Verification items for the finished model (mm, model axes). A direction names the side the tool comes from. Round coordinates to 2 decimals unless told otherwise and drop trailing zeros. Write each loop counter-clockwise with the first axis right and the second up, starting at its lowest first coordinate (ties: lowest second). Pieces come first, ordered by that corner, then holes. Notation, with made-up numbers: M 32,50.5 L 45,50.5 A23 ccw 45,69.5 Z; hole C -21.5,78.5 d6. An arc over 180 degrees is marked long. One line per question, with ' | ' between items. Start each with the question number.
Q1. Cross-section at B-B (y = -9.25). Record the boundary of the cut face in (x, z), then the cut area to 3 significant figures.
Q2. Tool access check on faces 1 (the face through (10.5, -6, 52)), 2 (the face through (-12, -5, 4)), 3 (the face through (-14, -3.5, 67)). Record the directions out of +Z, -Z, +X, -X, +Y, -Y that give a thin tool (end or side, any length) a straight path to the whole face; none if there is none.
Q3. Cross-section at A-A (x = -3.5). Record the boundary of the cut face in (y, z), then the cut area to 3 significant figures.
Q4. Gauge pin test, flat ends, axial feed: pin 1 (10 mm diameter, centred on x = 7, z = 36.5, fed in from -Y); pin 2 (4 mm diameter, centred on x = 1, z = 97, fed in from +Y); pin 3 (6 mm diameter, centred on x = -5.5, y = 9.5, fed in from +Z). Record the tip position at first contact, or that the pin passes through.
Q5. Thickness scan on line 1 along Y through (x, z) = (-10, 24); line 2 along Z through (x, y) = (7.25, 3.5); line 3 along X through (y, z) = (-6.5, 30). Record the ranges inside material, lowest first. Write a range as from..to.
from build123d import *

# Parameters (mm, degrees)
CROQUIS1_W              = 29
CROQUIS1_H              = 18
SALIENTE_EXTRUIR1_DEPTH = 4
CROQUIS2_W              = 6
CROQUIS2_H              = 4
CROQUIS2_W_2            = 9
SALIENTE_EXTRUIR3_DEPTH = 4
CROQUIS4_W              = 4.5
CROQUIS4_H              = 4
SALIENTE_EXTRUIR4_DEPTH = 100
CROQUIS5_W              = 7
CROQUIS5_H              = 4
SALIENTE_EXTRUIR5_DEPTH = 100
CROQUIS6_W              = 30
CROQUIS6_H              = 4
SALIENTE_EXTRUIR6_DEPTH = 10
CORTAR_EXTRUIR2_DEPTH   = 10
CORTAR_EXTRUIR3_DEPTH   = 10
CORTAR_EXTRUIR4_DEPTH   = 10
CORTAR_EXTRUIR5_DEPTH   = 10


with BuildPart() as part:
    # Croquis1 → Saliente-Extruir1 (new body)
    with BuildSketch(Plane(origin=(0, 0, 0), x_dir=(0, 1, 0), z_dir=(0, 0, 1))):
        Rectangle(CROQUIS1_W, CROQUIS1_H)
    extrude(amount=SALIENTE_EXTRUIR1_DEPTH)

    # Croquis2 → Saliente-Extruir3 (add)
    with BuildSketch(Plane.XY.offset(4)):
        with Locations((-12, -5.5)):
            Rectangle(CROQUIS2_W, CROQUIS2_H)
        with Locations((-4.5, -5.5)):
            Rectangle(CROQUIS2_W_2, CROQUIS2_H)
        with Locations((4.5, -5.5)):
            Rectangle(CROQUIS2_W_2, CROQUIS2_H)
        with Locations((12, -5.5)):
            Rectangle(CROQUIS2_W, CROQUIS2_H)
    extrude(amount=SALIENTE_EXTRUIR3_DEPTH)

    # Croquis4 → Saliente-Extruir4 (add)
    with BuildSketch(Plane.XY.offset(8)):
        with Locations((12.75, -5.5)):
            Rectangle(CROQUIS4_W, CROQUIS4_H)
    extrude(amount=SALIENTE_EXTRUIR4_DEPTH)

    # Croquis5 → Saliente-Extruir5 (add)
    with BuildSketch(Plane.XY.offset(8)):
        with Locations((-11.5, -5.5)):
            Rectangle(CROQUIS5_W, CROQUIS5_H)
    extrude(amount=SALIENTE_EXTRUIR5_DEPTH)

    # Croquis6 → Saliente-Extruir6 (add)
    with BuildSketch(Plane.XY.offset(108)):
        with Locations((0, -5.5)):
            Rectangle(CROQUIS6_W, CROQUIS6_H)
    extrude(amount=-SALIENTE_EXTRUIR6_DEPTH)

    # Croquis7 → Cortar-Extruir2 (cut)
    with BuildSketch(Plane.XZ.offset(7.5)):
        Polygon((-8, 96.258476268), (-8, 97.519571135), (-11.46482967, 97.519571135), align=None)
    extrude(amount=-CORTAR_EXTRUIR2_DEPTH, mode=Mode.SUBTRACT)

    # Croquis8 → Cortar-Extruir3 (cut)
    with BuildSketch(Plane(origin=(0, -7.5, 0), x_dir=(-1, 0, 0), z_dir=(0, -1, 0))):
        Polygon((8, -94.994476268), (11.46482967, -93.733381401), (8, -93.733381401), align=None)
    extrude(amount=-CORTAR_EXTRUIR3_DEPTH, mode=Mode.SUBTRACT)

    # Croquis9 → Cortar-Extruir4 (cut)
    with BuildSketch(Plane(origin=(0, -7.5, 0), x_dir=(-1, 0, 0), z_dir=(0, -1, 0))):
        Polygon((11.46482967, -93.733381401), (11.46482967, -92.469381401), (8, -91.208286534), (8, -93.733381401), align=None)
    extrude(amount=-CORTAR_EXTRUIR4_DEPTH, mode=Mode.SUBTRACT)

    # Croquis10 → Cortar-Extruir5 (cut)
    with BuildSketch(Plane(origin=(0, -3.5, 0), x_dir=(-1, 0, 0), z_dir=(0, 1, 0))):
        Polygon((11.46482967, 11.070269037), (8, 9.80917417), (8, 13.595363904), (11.46482967, 12.334269037), align=None)
        Polygon((11.46482967, 88.087115043), (8, 89.348209909), (8, 85.562020176), (11.46482967, 86.823115043), align=None)
        Polygon((8, 84.298020176), (11.46482967, 83.036925309), (11.46482967, 81.772925309), (8, 80.511830442), align=None)
        Polygon((8, 79.247830442), (11.46482967, 77.986735575), (11.46482967, 76.722735575), (8, 75.461640708), align=None)
        Polygon((8, 70.411450974), (8, 74.197640708), (11.46482967, 72.936545841), (11.46482967, 71.672545841), align=None)
        Polygon((8, 65.361261241), (8, 69.147450974), (11.46482967, 67.886356108), (11.46482967, 66.622356108), align=None)
        Polygon((8, 60.311071507), (8, 64.097261241), (11.46482967, 62.836166374), (11.46482967, 61.572166374), align=None)
        Polygon((8, 55.260881773), (8, 59.047071507), (11.46482967, 57.78597664), (11.46482967, 56.52197664), align=None)
        Polygon((8, 50.21069204), (8, 53.996881773), (11.46482967, 52.735786906), (11.46482967, 51.471786906), align=None)
        Polygon((8, 45.160502306), (8, 48.94669204), (11.46482967, 47.685597173), (11.46482967, 46.421597173), align=None)
        Polygon((8, 43.896502306), (11.46482967, 42.635407439), (11.46482967, 41.371407439), (8, 40.110312572), align=None)
        Polygon((8, 38.846312572), (8, 35.060122838), (11.46482967, 36.321217705), (11.46482967, 37.585217705), align=None)
        Polygon((8, 33.796122838), (8, 30.009933105), (11.46482967, 31.271027972), (11.46482967, 32.535027972), align=None)
        Polygon((8, 24.959743371), (8, 28.745933105), (11.46482967, 27.484838238), (11.46482967, 26.220838238), align=None)
        Polygon((8, 23.695743371), (8, 19.909553637), (11.46482967, 21.170648504), (11.46482967, 22.434648504), align=None)
        Polygon((8, 14.859363904), (8, 18.645553637), (11.46482967, 17.38445877), (11.46482967, 16.12045877), align=None)
    extrude(amount=-CORTAR_EXTRUIR5_DEPTH, mode=Mode.SUBTRACT)


solid = part.part
Determined:
1) outline: M -9,0 L 9,0 L 9,4 L -9,4 Z | area: 72.0 mm²
2) face 1: +Y, -Y | face 2: -Z, -X, +Y, -Y | face 3: +Z, +X, -X, +Y
3) outline: M -14.5,0 L 14.5,0 L 14.5,4 L -3.5,4 L -3.5,8 L -7.5,8 L -7.5,4 L -14.5,4 Z; M -7.5,98 L -3.5,98 L -3.5,108 L -7.5,108 Z | area: 172 mm²
4) pin 1: stops at y = -7.5 | pin 2: stops at y = -3.5 | pin 3: stops at z = 4
5) line 1: y = -7.5..-3.5 | line 2: z = 0..4 | line 3: x = -15..-8, 10.5..15
